```python
from build123d import *

# Parameters (mm, degrees)
BOSS_EXTRUDE1_DEPTH         = 12.5
SKETCH2_W                   = 5
SKETCH2_H                   = 35
BOSS_EXTRUDE2_DEPTH         = 17.5
TAP_DRILL_FOR_M3X0_5_TAP1_D = 2.5
RIB1_REACH                  = 57.79
SKETCH5_WALL_W              = 127.721703646
SKETCH5_WALL_H              = 10
RIB6_REACH                  = 57.79
SKETCH7_WALL_W              = 127.721703646
SKETCH7_WALL_H              = 10


with BuildPart() as part:
    # Sketch1 → Boss-Extrude1 (new, symmetric)
    with BuildSketch(Plane.XY):
        Polygon((-50, 17.5), (-50, -17.5), (-45, -17.5), (-45, -7.5), (50, -7.5), (50, 7.5), (-45, 7.5), (-45, 17.5), align=None)
    extrude(amount=BOSS_EXTRUDE1_DEPTH, both=True)

    # Sketch2 → Boss-Extrude2 (add, symmetric)
    with BuildSketch(Plane.XY):
        with Locations((-47.5, 0)):
            Rectangle(SKETCH2_W, SKETCH2_H)
    extrude(amount=BOSS_EXTRUDE2_DEPTH, both=True)

    # Tap Drill for M3x0.5 Tap1 (through all)
    with Locations(Plane.ZY.offset(50)):
        with Locations((-15, 13.5), (15, 13.5), (15, -13.5), (-15, -13.5)):
            Hole(TAP_DRILL_FOR_M3X0_5_TAP1_D / 2)

    # Sketch5 wall → Rib1 (add, up to next)
    with BuildSketch(Plane(origin=(-40, 12.5, 0), x_dir=(0.707106781187, -0.707106781187, 0), z_dir=(0.707106781187, 0.707106781187, 0)), mode=Mode.PRIVATE) as rib1_sk1:
        Rectangle(SKETCH5_WALL_W, SKETCH5_WALL_H)
    rib1_tool1 = extrude(rib1_sk1.sketch, amount=-RIB1_REACH, mode=Mode.PRIVATE) - part.part
    add(rib1_tool1.solids().sort_by_distance((-40, 12.5, 0))[0])

    # Sketch7 wall → Rib6 (add, up to next)
    with BuildSketch(Plane(origin=(-40, -12.5, 0), x_dir=(0.707106781187, 0.707106781187, 0), z_dir=(-0.707106781187, 0.707106781187, 0)), mode=Mode.PRIVATE) as rib6_sk1:
        Rectangle(SKETCH7_WALL_W, SKETCH7_WALL_H)
    rib6_tool1 = extrude(rib6_sk1.sketch, amount=RIB6_REACH, mode=Mode.PRIVATE) - part.part
    add(rib6_tool1.solids().sort_by_distance((-40, -12.5, 0))[0])


solid = part.part
```
Here's how the part is built. I have some questions about the finished solid (model axes, mm). A direction names the side the tool comes from. Give positions to 0.01 mm unless a question says otherwise; leave off trailing zeros. Order: outer loops, then holes, each group sorted by start corner. A loop starts at its lowest first (then second) coordinate and runs counter-clockwise, first axis right, second up. Notation, with made-up numbers: M 72.25,45.5 L 76.25,45.5 A35 cw 76.25,78.5 Z; hole C 40.5,21 d11. An arc over 180 degrees is marked long. Use a Markdown table: item, result. Add a question column.
1. Suppose I cut it at D-D (z = 0). List the corners of the cut face in (x, y) for me, and give its area (3 significant figures).
2. I need wall thicknesses on probe 1 along Y at (x, z) = (-48.35, 15); probe 2 along Z at (x, y) = (-48, 13); probe 3 along X at (y, z) = (-12.5, -9.5). Which ranges of each line are inside material? Lowest first, please. Write a range as from..to.
3. On a 3-axis mill with a long thin cutter (end or side, diameter ignored), from which of +Z, -Z, +X, -X, +Y, -Y can I reach the whole of each face in a straight line? I mean faces 1 (the flat face through (-42, -11, 5)), 2 (the flat face through (-48, 17.5, 0)), 3 (the flat face through (-42, -11, -5)), 4 (the flat face through (2, 0, 12.5)), 5 (the flat face through (2, 0, -12.5)). Say none if no direction works.
4. Suppose I cut it at B-B (z = -15). List the corners of the cut face in (x, y) for me, and give its area (3 significant figures).
5. Suppose I cut it at A-A (y = -13.5). List the corners of the cut face in (x, z) for me.
6. For pin 1 Ø12 at (x, y) = (-7, -3) entering from +Z; pin 2 Ø1.5 at (y, z) = (13.5, 15) entering from -X; pin 3 Ø3 at (x, z) = (27.5, -2) entering from -Y; pin 4 Ø2 at (x, z) = (-28, 8) entering from +Y, each with a flat end and sliding along its axis, tell me the tip position at first contact or that it passes through.
7. Suppose I cut it at C-C (x = 27). List the corners of the cut face in (y, z) for me.
8. If we mould it in two halves opening along Y, with no side actions, what happens to faces 6 (the cylindrical face through (-47.47, 14.74, -14.84)), 7 (the flat face through (3, 7.5, 0)), 8 (the flat face through (-48, 0, 17.5))? For each: +Y half, -Y half, draft (parallel to the pull), parting line (faces both ways), or undercut.
Results list:
| question | item | result |
|---|---|---|
| 1 | outline | M -50,-17.5 L -45,-17.5 L -35,-7.5 L 50,-7.5 L 50,7.5 L -35,7.5 L -45,17.5 L -50,17.5 Z |
| 1 | area | 1,700 mm² |
| 2 | probe 1 | y = -17.5..-14.75, -12.25..12.25, 14.75..17.5 |
| 2 | probe 2 | z = -17.5..-16.15, -13.85..13.85, 16.15..17.5 |
| 2 | probe 3 | x = -50..-45 |
| 3 | face 1 | +Z, +X, -Y |
| 3 | face 2 | +Z, -Z, +X, -X, +Y |
| 3 | face 3 | -Z, +X, -Y |
| 3 | face 4 | +Z, +X, +Y, -Y |
| 3 | face 5 | -Z, +X, +Y, -Y |
| 4 | outline | M -50,-17.5 L -45,-17.5 L -45,-14.75 L -50,-14.75 Z; M -50,-12.25 L -45,-12.25 L -45,12.25 L -50,12.25 Z; M -50,14.75 L -45,14.75 L -45,17.5 L -50,17.5 Z |
| 4 | area | 150 mm² |
| 5 | outline | M -50,-17.5 L -45,-17.5 L -45,-16.25 L -50,-16.25 Z; M -50,-13.75 L -45,-13.75 L -45,-5 L -41,-5 L -41,5 L -45,5 L -45,13.75 L -50,13.75 Z; M -50,16.25 L -45,16.25 L -45,17.5 L -50,17.5 Z |
| 6 | pin 1 | stops at z = 12.5 |
| 6 | pin 2 | passes through |
| 6 | pin 3 | stops at y = -7.5 |
| 6 | pin 4 | stops at y = 7.5 |
| 7 | outline | M -7.5,-12.5 L 7.5,-12.5 L 7.5,12.5 L -7.5,12.5 Z |
| 8 | face 6 | undercut |
| 8 | face 7 | +Y half |
| 8 | face 8 | draft |
